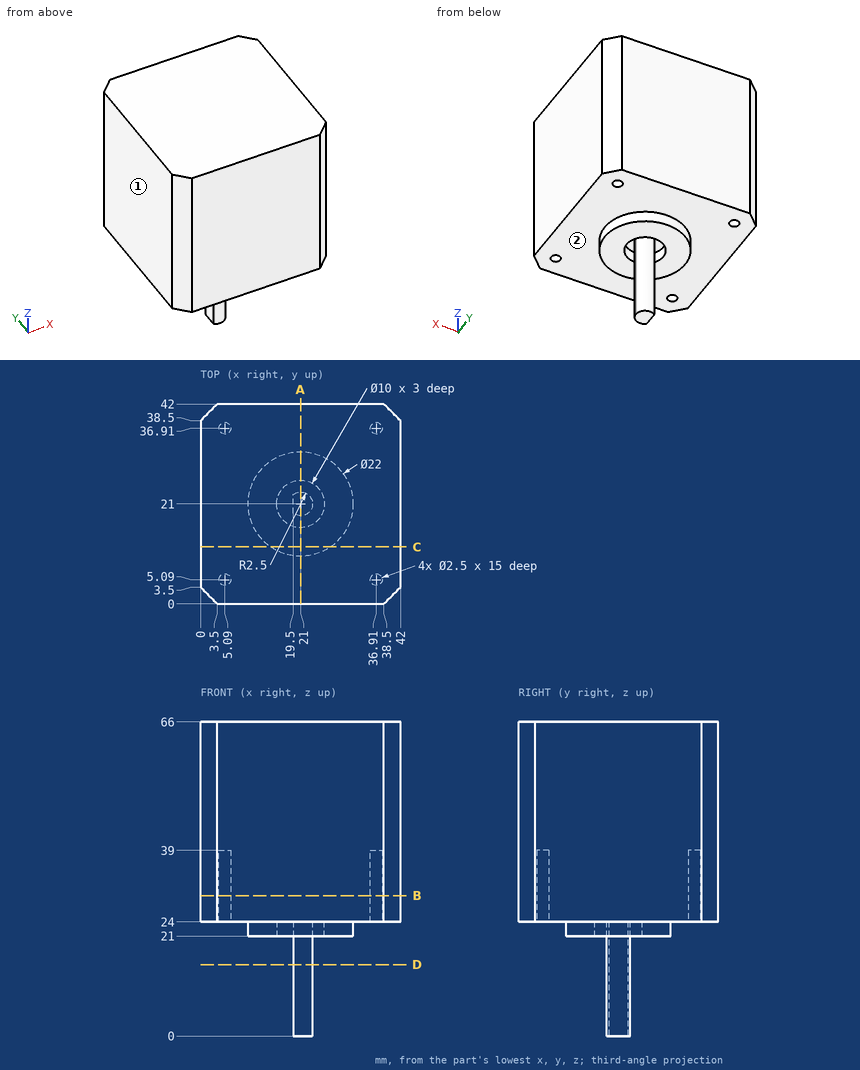
Verification items for this drawing (mm, ordinates from the low corner). A direction names the side the tool comes from. Coordinates: 2 decimals unless noted, no trailing zeros. Order: outer loops, then holes, each group sorted by start corner. A loop starts at its lowest first (then second) coordinate and runs counter-clockwise, first axis right, second up. Notation, with made-up numbers: (38.5, 24) - (53.5, 24) arc R30 ccw to (53.5, 46) - close; hole circle Ø7 at (85, -0.5). An arc over 180 degrees is marked (long way). Use one line per item in the form item = value.
1. Gauge pin test, flat ends, axial feed: pin 1 (3 mm diameter, centred on x = 5, y = 5, fed in from -Z); pin 2 (0.8 mm diameter, centred on x = 5, y = 36.5, fed in from -Z); pin 3 (3 mm diameter, centred on y = 21.5, z = 12.5, fed in from -X); pin 4 (6 mm diameter, centred on x = 36, z = 19, fed in from +Y). Record the tip position at first contact, or that the pin passes through.
Here are the results:
pin_1 = 24
pin_2 = 39
pin_3 = 19.5
pin_4 = through
2. Scan lines: line 1 (Y direction, x = 21, z = 22); line 2 (X direction, y = 38, z = 26.5); line 3 (Z direction, x = 9.5, y = 16.5). Record each from-to range of solid material in increasing order.
Here are the results:
line_1 = 10 to 16, 18.5 to 23.5, 26 to 32
line_2 = 0 to 4.48, 5.7 to 36.3, 37.52 to 42
line_3 = 24 to 66
3. Access from +Z, -Z, +X, -X, +Y, -Y to the whole of each face (thin tool, end or side, straight path). Record for the marked faces 1 and 2.
Here are the results:
face_1 = +Z, -Z, -X, +Y, -Y
face_2 = -Z
4. Section check B-B (z = 29.5). Record the boundary of the cut face in (x, y), then the cut area to 3 significant figures.
Here are the results:
outline = (0, 3.5) - (3.5, 0) - (38.5, 0) - (42, 3.5) - (42, 38.5) - (38.5, 42) - (3.5, 42) - (0, 38.5) - close; hole circle Ø2.5 at (5.09, 5.09); hole circle Ø2.5 at (5.09, 36.91); hole circle Ø2.5 at (36.91, 5.09); hole circle Ø2.5 at (36.91, 36.91)
area = 1,720 mm²
5. Section check C-C (y = 12). Record the boundary of the cut face in (x, z).
Here are the results:
outline = (0, 24) - (14.68, 24) - (14.68, 21) - (27.32, 21) - (27.32, 24) - (42, 24) - (42, 66) - (0, 66) - close
6. Section check D-D (z = 15). Record the boundary of the cut face in (x, y), then the cut area to 3 significant figures.
Here are the results:
outline = (19.5, 19) arc R2.5 ccw (long way) to (19.5, 23) - close
area = 16.8 mm²
7. Section check A-A (x = 21). Record the boundary of the cut face in (y, z).
Here are the results:
outline = (0, 24) - (10, 24) - (10, 21) - (16, 21) - (16, 24) - (18.5, 24) - (18.5, 0) - (23.5, 0) - (23.5, 24) - (26, 24) - (26, 21) - (32, 21) - (32, 24) - (42, 24) - (42, 66) - (0, 66) - close
